```python
from build123d import *

# Parameters (mm, degrees)
SKETCH1_W           = 76.2
SKETCH1_H           = 44.45
BOSS_EXTRUDE1_DEPTH = 6.35
FILLET1_R           = 6.35
SKETCH2_R           = 2.4892
SKETCH2_R_2         = 10.025399939
CUT_EXTRUDE1_DEPTH  = 7.35


with BuildPart() as part:
    # Sketch1 → Boss-Extrude1 (new body)
    with BuildSketch(Plane(origin=(0, 0, 0), x_dir=(1, 0, 0), z_dir=(0, 1, 0))):
        with Locations((38.1, 22.225)):
            Rectangle(SKETCH1_W, SKETCH1_H)
    extrude(amount=BOSS_EXTRUDE1_DEPTH)

    # Fillet1
    fillet1_edges = [part.edges().sort_by_distance(p)[0] for p in [
        (0, 3.175, -44.45),
        (76.2, 3.175, -44.45),
        (76.2, 3.175, 0),
        (0, 3.175, 0),
    ]]
    fillet(fillet1_edges, radius=FILLET1_R)

    # Sketch2 → Cut-Extrude1 (cut, through all)
    with BuildSketch(Plane(origin=(0, 6.35, 0), x_dir=(1, 0, 0), z_dir=(0, 1, 0))):
        with Locations((31.75, 34.925)):
            Circle(SKETCH2_R)
        with Locations((6.35, 34.925)):
            Circle(SKETCH2_R)
        with Locations((19.05, 34.925)):
            Circle(SKETCH2_R)
        with Locations((19.05, 22.225)):
            Circle(SKETCH2_R)
        with Locations((6.35, 22.225)):
            Circle(SKETCH2_R)
        with Locations((6.35, 9.525)):
            Circle(SKETCH2_R)
        with Locations((19.05, 9.525)):
            Circle(SKETCH2_R)
        with Locations((31.75, 9.525)):
            Circle(SKETCH2_R)
        with Locations((57.15, 9.525)):
            Circle(SKETCH2_R)
        with Locations((69.85, 9.525)):
            Circle(SKETCH2_R)
        with Locations((69.85, 22.225)):
            Circle(SKETCH2_R)
        with Locations((69.85, 34.925)):
            Circle(SKETCH2_R)
        with Locations((57.15, 34.925)):
            Circle(SKETCH2_R)
        with Locations((44.45, 22.225)):
            Circle(SKETCH2_R_2)
    extrude(amount=-CUT_EXTRUDE1_DEPTH, mode=Mode.SUBTRACT)


solid = part.part
```
Design review of the part built by this model. Coordinates are the model's own, in mm. Give positions to 0.01 mm unless a question says otherwise; leave off trailing zeros. Order: outer loops, then holes, each group sorted by start corner. A loop starts at its lowest first (then second) coordinate and runs counter-clockwise, first axis right, second up. Notation, with made-up numbers: (9.25, 25.25) -> (37.25, 25.25) arc R22 cw to (37.25, 61.25) -> close; hole circle Ø4 at (61, -32.5). An arc over 180 degrees is marked (long way). Write each question's results on one line, items separated by ' | '. Start each with the question number.
Q1. Add section C-C on x = 19.05. Give the boundary of the cut face in (y, z).
Q2. Wall thickness on L1, parallel to Z at x = 57.15, y = 3; L2, parallel to X at y = 5.5, z = -11; L3, parallel to X at y = 2, z = -34: over which ranges is each line inside the solid? List them lowest first. Write a range as from..to.
Q3. Add section B-B on z = -30. Give the boundary of the cut face in (x, y), and give its area (3 significant figures).
Q4. Mouldability with a two-part tool opening along Z and no side actions: class faces 1 (the flat face through (38, 3, 0)), 2 (the flat face through (38, 3, -44.45)), 3 (the cylindrical face through (18.726, 3.219, -37.393)) as +Z half, -Z half, draft (parallel to the pull), parting line (faces both ways), or undercut.
Q5. Add section A-A on x = 44.45. Give the boundary of the cut face in (y, z).
Q6. Add section D-D on y = 5.25. State how many separate pieces and enclosed holes the cut face has, and give its area (3 significant figures).
Found:
1) outline: (0, -44.45) -> (6.35, -44.45) -> (6.35, -37.41) -> (0, -37.41) -> close; (0, -32.44) -> (6.35, -32.44) -> (6.35, -24.71) -> (0, -24.71) -> close; (0, -19.74) -> (6.35, -19.74) -> (6.35, -12.01) -> (0, -12.01) -> close; (0, -7.04) -> (6.35, -7.04) -> (6.35, 0) -> (0, 0) -> close
2) L1: z = -44.45..-37.41, -32.44..-12.01, -7.04..0 | L2: x = 0..4.34, 8.36..17.04, 21.06..29.74, 33.76..55.14, 59.16..67.84, 71.86..76.2 | L3: x = 0..4.04, 8.66..16.74, 21.36..29.44, 34.06..54.84, 59.46..67.54, 72.16..76.2
3) outline: (0, 0) -> (38.12, 0) -> (38.12, 6.35) -> (0, 6.35) -> close; (50.78, 0) -> (76.2, 0) -> (76.2, 6.35) -> (50.78, 6.35) -> close | area: 403 mm2
4) face 1: +Z half | face 2: -Z half | face 3: undercut
5) outline: (0, -44.45) -> (6.35, -44.45) -> (6.35, -32.25) -> (0, -32.25) -> close; (0, -12.2) -> (6.35, -12.2) -> (6.35, 0) -> (0, 0) -> close
6) separate pieces: 1 | enclosed holes: 14 | area: 2,780 mm2
